CAD build for the part. Positions are in the model's coordinates, mm. Face numbers are marked on the shaded views. A direction names the side the tool comes from. Coordinates: 2 decimals unless noted, no trailing zeros. Loops run counter-clockwise (first coordinate to the right, second up) from the corner with the lowest first, then second, coordinate; pieces in that order, holes last. Notation, with made-up numbers: (13.5, -24.5) -> (31.5, -24.5) arc R33 ccw to (31.5, 4.5) -> close; hole circle Ø11 at (23.25, 32.5). An arc over 180 degrees is marked (long way). Answer as a JSON object with one key per item and string values. Group by question number.
from build123d import *

# Parameters (mm, degrees)
F1_DEPTH      = 12.7
F2_R          = 3.175
F3_DEPTH      = 3.175
F4_R          = 3.175
F5_DEPTH      = 3.175
F6_R          = 3.175
F7_DEPTH      = 25.4
F7_DEPTH_BACK = 25.4


with BuildPart() as f1:
    # F0 (on Front) → F1 (new body)
    with BuildSketch(Plane.XZ):
        with BuildLine():
            Line((-8.097896, -4.769327), (8.097896, -4.769327))
            ThreePointArc((8.097896, -4.769327), (0, 9.398), (-8.097896, -4.769327))
        make_face()
    extrude(amount=F1_DEPTH)

    # F2 (on face) → F3 (join)
    with BuildSketch(Plane.XZ.offset(12.7)):
        Circle(F2_R)
    extrude(amount=F3_DEPTH)

    # F4 (on face) → F5 (join)
    with BuildSketch(Plane(origin=(0, 0, 0), x_dir=(-1, 0, 0), z_dir=(0, 1, 0))):
        Circle(F4_R)
    extrude(amount=F5_DEPTH)

    # F6 (on face) → F7 (cut, two sides)
    with BuildSketch(Plane(origin=(0, 0, -4.769327), x_dir=(1, 0, 0), z_dir=(0, 0, -1))) as f7_sk:
        with Locations((0, 6.35)):
            Circle(F6_R)
    extrude(amount=-F7_DEPTH, mode=Mode.SUBTRACT)
    extrude(f7_sk.sketch, amount=-F7_DEPTH_BACK, mode=Mode.SUBTRACT)


solid = f1.part
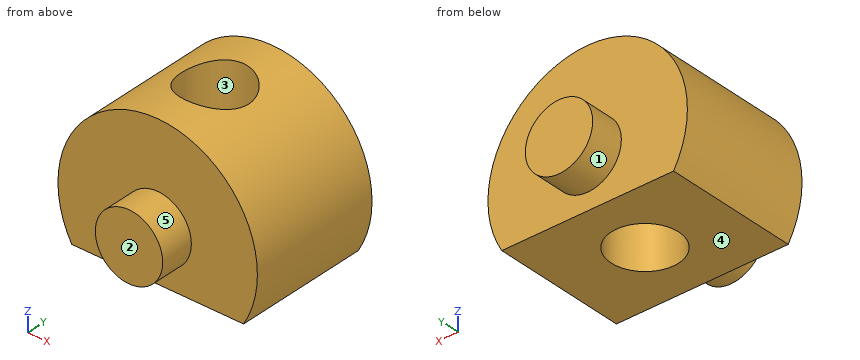
Item 1: Band-saw the part on B-B, the plane z = 0. List the corners of the cut face in (x, y) (3 decimals).
Item 2: Drill centre lines: L1, parallel to Y at x = 0, z = 3.75 (3 decimals); L2, parallel to Y at x = 6.25, z = 0.25; L3, parallel to Y at x = 0, z = 0.5 (3 decimals). Where is each one in solid material? Low to high.
Item 3: Band-saw the part on D-D, the plane y = -13.5. List the corners of the cut face in (x, z) (3 decimals), and give its area (3 significant figures).
Item 4: Pull direction X, two halves, no side cores. Call the marked faces 3, 4 and 5: +X half, -X half, draft (parallel to the pull), parting line (faces both ways), or undercut.
Item 5: Band-saw the part on C-C, the plane y = -6.35. List the corners of the cut face in (x, z) (3 decimals).
Item 6: 3-axis set-ups, long thin cutter, end or side, ignore diameter. For the marked faces 1 and 2: which of +Z, -Z, +X, -X, +Y, -Y reach the whole face in a straight line?
Item 7: Flat gauge pins, fed straight in: P1, Ø8, axis at y = -7.5, z = 7, coming from the -X side; P2, Ø1, axis at x = -5, z = -3, coming from the +Y side; P3, Ø2, axis at x = -1.5, y = -13, coming from the +Z side. Where does each tip first touch, or does it go through?
Item 8: Band-saw the part on A-A, the plane x = 0. List the corners of the cut face in (y, z) (3 decimals).
Reply:
{
 "1": {"outline": "(-9.398, -12.7) -> (-3.175, -12.7) -> (-3.175, -15.875) -> (3.175, -15.875) -> (3.175, -12.7) -> (9.398, -12.7) -> (9.398, 0) -> (3.175, 0) -> (3.175, 3.175) -> (-3.175, 3.175) -> (-3.175, 0) -> (-9.398, 0) -> close; hole circle Ø6.35 at (0, -6.35)"},
 "2": {"L1": "-12.7 to -9.525, -3.175 to 0", "L2": "-12.7 to 0", "L3": "-15.875 to -9.525, -3.175 to 3.175"},
 "3": {"outline": "circle Ø6.35 at (0, 0)", "area": "31.7 mm²"},
 "4": {"face 3": "undercut", "face 4": "draft", "face 5": "parting line"},
 "5": {"outline": "(-8.098, -4.769) -> (-3.175, -4.769) -> (-3.175, 8.845) arc R9.398 ccw to start; (3.175, -4.769) -> (8.098, -4.769) arc R9.398 ccw to (3.175, 8.845) -> close"},
 "6": {"face 1": "+Y", "face 2": "+Z, -Z, +X, -X, -Y"},
 "7": {"P1": "x = -8.91", "P2": "y = 0", "P3": "z = 9.38"},
 "8": {"outline": "(-15.875, -3.175) -> (-12.7, -3.175) -> (-12.7, -4.769) -> (-9.525, -4.769) -> (-9.525, 9.398) -> (-12.7, 9.398) -> (-12.7, 3.175) -> (-15.875, 3.175) -> close; (-3.175, -4.769) -> (0, -4.769) -> (0, -3.175) -> (3.175, -3.175) -> (3.175, 3.175) -> (0, 3.175) -> (0, 9.398) -> (-3.175, 9.398) -> close"}
}
